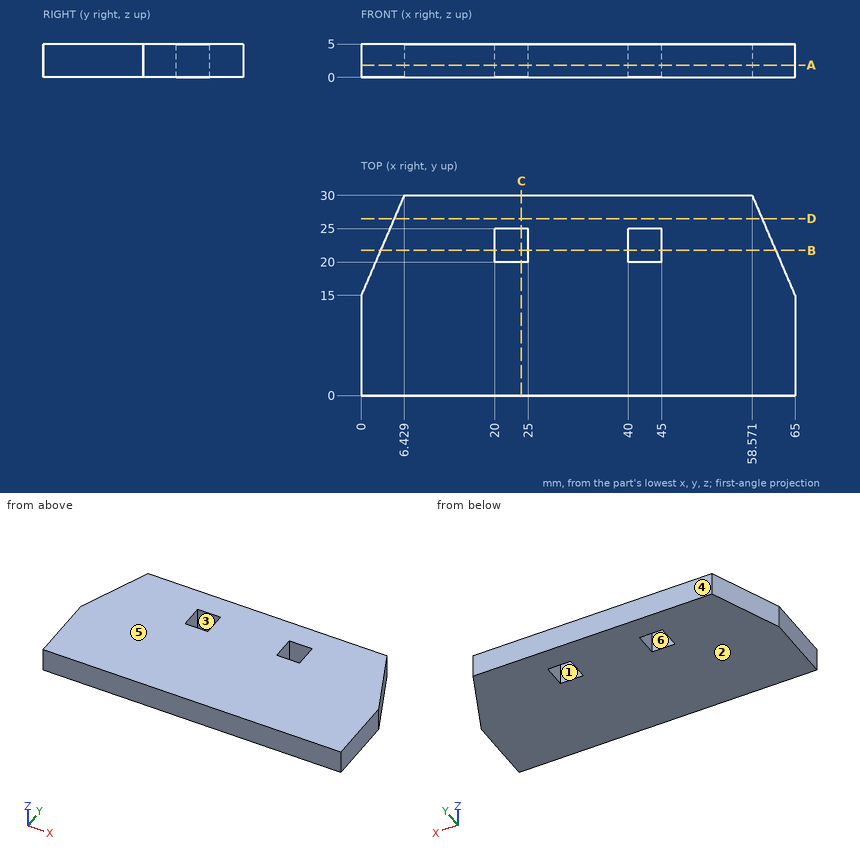
Geometry check sheet. Reference: drawing and pictorial views, mm from the part's lowest x, y, z. A direction names the side the tool comes from. Coordinates: 2 decimals unless noted, no trailing zeros. Order: outer loops, then holes, each group sorted by start corner. A loop starts at its lowest first (then second) coordinate and runs counter-clockwise, first axis right, second up.
Item 1: Mould release check, pull along Y, two halves, no side actions. Record for the marked faces 3, 4, 5 and 6: released by +Y, released by -Y, zero draft, split by the parting line, or undercut.
Item 2: Tool access check on the marked faces 1 and 2. Record the directions out of +Z, -Z, +X, -X, +Y, -Y that give a thin tool (end or side, any length) a straight path to the whole face; none if there is none.
Item 3: Depth check by flat-ended pin: pin 1 (2.5 mm diameter, centred on y = 22.5, z = 2, fed in from -X); pin 2 (2.5 mm diameter, centred on y = 23.5, z = 2, fed in from -X); pin 3 (1.5 mm diameter, centred on y = 17, z = 3.5, fed in from +X) (1 decimal). Enter the tip coordinate at first touch or a pass-through.
Item 4: Scan lines: line 1 along Y through (x, z) = (23.5, 4.2); line 2 along X through (y, z) = (23.5, 1.25); line 3 along X through (y, z) = (20.75, 2.05) (1 decimal). Record each from-to range of solid material in increasing order.
Item 5: Section check D-D (y = 26.5). Enter the section's corners in (x, z), plus the area to 3 significant figures.
Item 6: Section check A-A (z = 1.85). Enter the section's corners in (x, y).
Item 7: Section check B-B (y = 21.75). Enter the section's corners in (x, z).
Item 8: Section check C-C (x = 24). Enter the section's corners in (y, z), plus the area to 3 significant figures.
Check sheet entries:
1. face 3: undercut
1. face 4: released by +Y
1. face 5: zero draft
1. face 6: undercut
2. face 1: +Z, -Z
2. face 2: -Z, +X, -X, +Y, -Y
3. pin 1: stops at x = 2.68
3. pin 2: stops at x = 3.11
3. pin 3: stops at x = 64.5
4. line 1: y = 0 to 20, 25 to 30
4. line 2: x = 3.64 to 20, 25 to 40, 45 to 61.36
4. line 3: x = 2.5 to 20, 25 to 40, 45 to 62.5
5. outline: (4.93, 0) - (60.07, 0) - (60.07, 5) - (4.93, 5) - close
5. area: 276 mm2
6. outline: (0, 0) - (65, 0) - (65, 15) - (58.57, 30) - (6.43, 30) - (0, 15) - close; hole (20, 20) - (25, 20) - (25, 25) - (20, 25) - close; hole (40, 20) - (45, 20) - (45, 25) - (40, 25) - close
7. outline: (2.89, 0) - (20, 0) - (20, 5) - (2.89, 5) - close; (25, 0) - (40, 0) - (40, 5) - (25, 5) - close; (45, 0) - (62.11, 0) - (62.11, 5) - (45, 5) - close
8. outline: (0, 0) - (20, 0) - (20, 5) - (0, 5) - close; (25, 0) - (30, 0) - (30, 5) - (25, 5) - close
8. area: 125 mm2
